from build123d import *

# Parameters (mm, degrees)
F1_DEPTH = 25.4
F2_R     = 6.35
F3_SIZE  = 6.35
F5_D     = 5.4102
F5_DEPTH = 19.05
F5_TIP   = 1.6253880605


with BuildPart() as f1:
    # F0 (on Front) → F1 (new body)
    with BuildSketch(Plane.XZ):
        Polygon((41.275, 42.8625), (-38.1, 42.8625), (-38.1, -33.3375), (41.275, -33.3375), (41.275, -17.4625), (-12.7, -17.4625), (-12.7, 17.4625), (41.275, 17.4625), align=None)
    extrude(amount=F1_DEPTH)

    # F2
    f2_edges = [f1.edges().sort_by_distance(p)[0] for p in [
        (-12.7, -12.7, 17.4625),
        (-12.7, -12.7, -17.4625),
    ]]
    fillet(f2_edges, radius=F2_R)

    # F3
    f3_edges = [f1.edges().sort_by_distance(p)[0] for p in [
        (41.275, -12.7, -17.4625),
        (41.275, -12.7, 17.4625),
    ]]
    chamfer(f3_edges, length=F3_SIZE)

    # F5
    with Locations(Plane.XY.offset(42.8625)):
        with Locations((15.875, -12.7)):
            Hole(F5_D / 2, depth=F5_DEPTH)
            with Locations((0, 0, -(F5_DEPTH + F5_TIP / 2))):  # 118° drill point
                Cone(0, F5_D / 2, F5_TIP, mode=Mode.SUBTRACT)


solid = f1.part
Read the model definition and answer for the solid it produces. Units are mm, in the model's axes. A direction names the side the tool comes from. Give positions to 0.01 mm unless a question says otherwise; leave off trailing zeros. Write each loop counter-clockwise with the first axis right and the second up, starting at its lowest first coordinate (ties: lowest second). Pieces come first, ordered by that corner, then holes. Notation, with made-up numbers: (-1, 13.5) -> (47, 13.5) arc R18 cw to (47, 37.5) -> close; hole circle Ø2 at (37, 54.5). An arc over 180 degrees is marked (long way). Answer as a JSON object with one key per item and string values. Group by question number.
1) Consider L1, parallel to Z at x = 2.5, y = -11.5; L2, parallel to X at y = -12.7, z = 34.25 (3 decimals); L3, parallel to Z at x = -9, y = -23. Determine where each line is inside the solid, lowest interval first. Write a range as from..to.
2) Find section B-B (z = -16). Write down the section's boundary in (x, y).
3) A tool of negligible diameter and unlimited length cuts with its end or side. For faces 1 (the cylindrical face through (13.295, -11.887, 33.204)), 2 (the flat face through (38.14, -12.52, 20.68)), 3 (the flat face through (-17, 0, 5)), from which of +Z, -Z, +X, -X, +Y, -Y can it reach the whole face along a straight path? Write none if from no direction.
4) The mould has two halves that part along Z. Classify faces 4 (the conical face through (15.53, -12.38, 22.47)), 5 (the flat face through (-38.1, -13, 5)), 6 (the flat face through (1, -13, -33.338)), 7 (the flat face through (15, -13, -17.462)): +Z half, -Z half, draft (parallel to the pull), parting line (faces both ways), or undercut.
Values follow:
{
 "1": {"L1": "z = -33.34..-17.46, 17.46..42.86", "L2": "x = -38.1..13.17, 18.58..41.275", "L3": "z = -33.34..-16.88, 16.88..42.86"},
 "2": {"outline": "(-38.1, -25.4) -> (-10.4, -25.4) -> (-10.4, 0) -> (-38.1, 0) -> close"},
 "3": {"face 1": "+Z", "face 2": "+X, +Y, -Y", "face 3": "+Z, -Z, +X, -X, +Y"},
 "4": {"face 4": "+Z half", "face 5": "draft", "face 6": "-Z half", "face 7": "undercut"}
}
